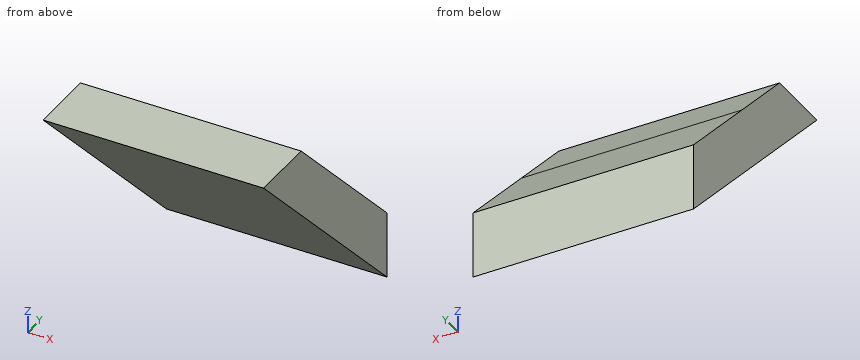
```python
from build123d import *

# Parameters (mm, degrees)
F0_W     = 85
F0_H     = 85
F1_DEPTH = 42.5
F7_DEPTH = 50


with BuildPart() as f1:
    # F0 (on Top) → F1 (new body, symmetric)
    with BuildSketch(Plane.XY):
        Rectangle(F0_W, F0_H)
    extrude(amount=F1_DEPTH, both=True)

    # F6 (on Right) → F7 (cut, symmetric)
    with BuildSketch(Plane.YZ):
        Polygon((75.503635, -75.503635), (0, 0), (-49.804213, 49.804213), (-49.804213, -75.503635), align=None)
        Polygon((-34.243761, 60.113393), (9.302937, 16.566695), (63.825734, -37.956103), (63.825734, 60.113393), align=None)
    extrude(amount=F7_DEPTH, both=True, mode=Mode.SUBTRACT)


solid = f1.part
```
CAD build for the part. Positions are in the model's coordinates, mm. Round coordinates to 2 decimals unless told otherwise and drop trailing zeros. Loops run counter-clockwise (first coordinate to the right, second up) from the corner with the lowest first, then second, coordinate; pieces in that order, holes last. Notation, with made-up numbers: (-2.5, 23) - (15.5, 23) arc R20 ccw to (15.5, 48) - close; hole circle Ø2 at (62, 49). An arc over 180 degrees is marked (long way). Return JSON: item names as keys, results as strings. Group by question number.
Q1. Band-saw the part on B-B on y = -20. Give the cut face in (x, z), plus the area to 3 significant figures.
Q2. Band-saw the part on C-C on z = -33.5. Give the cut face in (x, y).
Q3. Drill centre lines: line 1 along Z through (x, y) = (20, 20); line 2 along Y through (x, z) = (-5.5, -11); line 3 along Z through (x, y) = (38.5, 28.5). Where is each one in solid material? Low to high. Write a range as [from, to].
Q4. Flat gauge pins, fed straight in: pin 1 Ø12 at (x, z) = (-13, 9) entering from +Y; pin 2 Ø2 at (x, y) = (4.5, 27.5) entering from +Z; pin 3 Ø6 at (x, z) = (18, 1) entering from +Y. Where does each tip first touch, or does it go through?
Q5. Band-saw the part on A-A on x = 18. Give the cut face in (y, z).
Solutions:
{
 "1": {"outline": "(-42.5, 20) - (42.5, 20) - (42.5, 42.5) - (-42.5, 42.5) - close", "area": "1,910 mm^2"},
 "2": {"outline": "(-42.5, 33.5) - (42.5, 33.5) - (42.5, 42.5) - (-42.5, 42.5) - close"},
 "3": {"line 1": "z = [-20, 5.87]", "line 2": "y = [11, 36.87]", "line 3": "z = [-28.5, -2.63]"},
 "4": {"pin 1": "stops at y = 22.87", "pin 2": "stops at z = -0.63", "pin 3": "stops at y = 27.87"},
 "5": {"outline": "(-42.5, 42.5) - (42.5, -42.5) - (42.5, -16.63) - (-16.63, 42.5) - close"}
}
